Autodesk Inventor part; units mm, degrees
ref_plane "YZ Plane" through (0, 0, 0) normal (1, 0, 0) x (0, 1, 0)
ref_plane "XZ Plane" through (0, 0, 0) normal (0, 1, 0) x (-1, 0, 0)
ref_plane "XY Plane" through (0, 0, 0) normal (0, 0, 1) x (1, 0, 0)
sketch "Sketch1" plane through (0, 0, 0) normal (0, 0, 1) x (1, 0, 0)
  line L0 (-200, -50) -> (200, -50)
  line L1 (200, -50) -> (200, 50)
  line L2 (200, 50) -> (-200, 50)
  line L3 (-200, 50) -> (-200, -50)
  line L4 (-200, -50) -> (200, 50) construction
  line L5 (200, -50) -> (-200, 50) construction
  point P0 (0, 0)
  dimension "d0" = 400
  dimension "d1" = 100
extrude "Extrusion1" add sketch "Sketch1" along normal blind 9.5 and the other way blind 9.5
sketch "Sketch2" plane through (0, 0, 9.5) normal (0, 0, 1) x (1, 0, 0)
  line L0 (-200, 50) -> (-200, -50)
  line L1 (-200, 0) -> (-150, 0)
  line L2 (200, -50) -> (200, 50)
  line L3 (200, 0) -> (150, 0)
  circle A0 centre (-150, 0) radius 4
  circle A1 centre (150, 0) radius 4
  point P0 (0, 0)
  dimension "d6" = 50
  dimension "d7" = 50
  dimension "d8" = 8
  dimension "d9" = 8
extrude "Extrusion2" cut sketch "Sketch2" against normal blind 11
sketch "Sketch3" plane through (200, -50, 9.5) normal (1, 0, 0) x (0, 0, -1)
  circle A0 centre (9.5, 50) radius 4
  dimension "d12" = 8
extrude "Extrusion3" cut sketch "Sketch3" against normal blind 11
sketch "Sketch4" plane through (-200, -50, 9.5) normal (-1, 0, 0) x (0, 0, 1)
  circle A0 centre (-9.5, 50) radius 4
  dimension "d15" = 8
extrude "Extrusion4" cut sketch "Sketch4" against normal blind 11
properties part number "A"
Here's how the part is built. I have some questions about the finished solid (model axes, mm). A direction names the side the tool comes from. Give positions to 0.01 mm unless a question says otherwise; leave off trailing zeros. Order: outer loops, then holes, each group sorted by start corner. A loop starts at its lowest first (then second) coordinate and runs counter-clockwise, first axis right, second up. Notation, with made-up numbers: (32.5, -1) -> (54.5, -1) arc R27 cw to (54.5, 29) -> close; hole circle Ø10 at (-17, 43.25). An arc over 180 degrees is marked (long way). Use CSV: the item, a comma, the result in double quotes. Start each with the question number.
Item 1: Suppose I cut it at A-A (x = -150). List the corners of the cut face in (y, z) for me, and give its area (3 significant figures).
Item 2: Thinking about a two-plate mould opening in Z: for faces 1 (the flat face through (-189, 0, 0)), 2 (the flat face through (-3, 1, -9.5)), 3 (the flat face through (150, 0, -1.5)), 4 (the cylindrical face through (194.577, -3.905, 0.867)), which applies, pulls with the +Z half, pulls with the -Z half, needs draft (parallel to the pull), parting line crosses it, or undercut?
Item 3: On a 3-axis mill with a long thin cutter (end or side, diameter ignored), from which of +Z, -Z, +X, -X, +Y, -Y can I reach the whole of each face in a straight line? I mean faces 5 (the cylindrical face through (-146.185, 1.201, 4.077)), 6 (the flat face through (189, 0, 0)), 7 (the cylindrical face through (-194.577, -3.905, -0.867)). Say none if no direction works.
Item 4: If I drill on probe 1 along Y at (x, z) = (150, 7.25), over which ranges is the centre line in solid material (lowest first)? Write a range as [from, to].
Item 5: I'm going to push flat-ended pins straight in: P1, Ø2.5, axis at y = 1, z = 1.5, coming from the +X side; P2, Ø10.5, axis at y = 0, z = 0, coming from the -X side; P3, Ø4, axis at x = 150, y = -0.5, coming from the +Z side. Where does each tip first touch, or does it pass through?
Item 6: Suppose I cut it at B-B (y = 0). List the corners of the cut face in (x, z) for me.
Answer block:
1,outline,"(-50, -9.5) -> (50, -9.5) -> (50, 9.5) -> (4, 9.5) -> (4, -1.5) -> (-4, -1.5) -> (-4, 9.5) -> (-50, 9.5) -> close"
1,area,"1,810 mm^2"
2,face 1,"undercut"
2,face 2,"pulls with the -Z half"
2,face 3,"pulls with the +Z half"
2,face 4,"undercut"
3,face 5,"+Z"
3,face 6,"+X"
3,face 7,"-X"
4,probe 1,"y = [-50, -4], [4, 50]"
5,P1,"stops at x = 189"
5,P2,"stops at x = -200"
5,P3,"stops at z = -1.5"
6,outline,"(-200, -9.5) -> (200, -9.5) -> (200, -4) -> (189, -4) -> (189, 4) -> (200, 4) -> (200, 9.5) -> (154, 9.5) -> (154, -1.5) -> (146, -1.5) -> (146, 9.5) -> (-146, 9.5) -> (-146, -1.5) -> (-154, -1.5) -> (-154, 9.5) -> (-200, 9.5) -> (-200, 4) -> (-189, 4) -> (-189, -4) -> (-200, -4) -> close"
